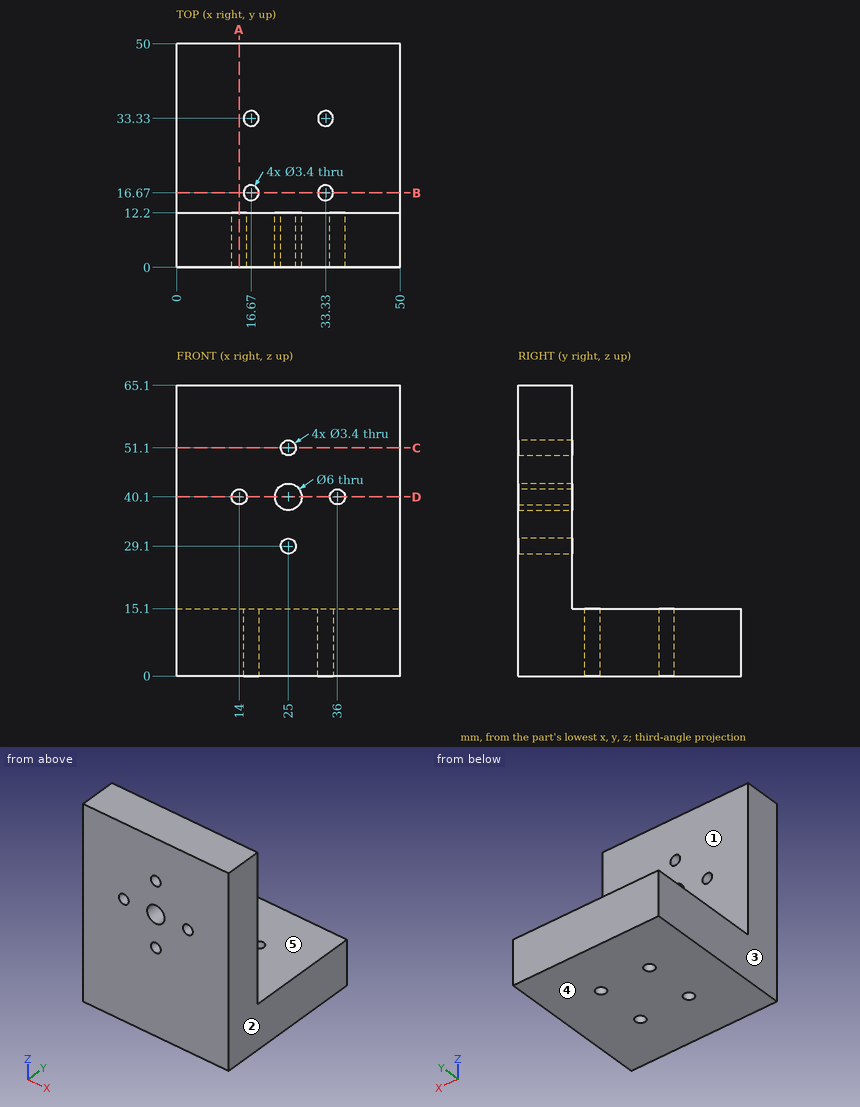
Geometry check sheet. Reference: drawing and pictorial views, mm from the part's lowest x, y, z. A direction names the side the tool comes from. Coordinates: 2 decimals unless noted, no trailing zeros. Write each loop counter-clockwise with the first axis right and the second up, starting at its lowest first coordinate (ties: lowest second). Pieces come first, ordered by that corner, then holes. Notation, with made-up numbers: (81.25, 37.25) -> (87.25, 37.25) arc R24 ccw to (87.25, 51.25) -> close; hole circle Ø8 at (63, 33). An arc over 180 degrees is marked (long way). Use a Markdown table: item, result.
1. Sectioned sample at D-D (z = 40.1). Enter the section's corners in (x, y), plus the area to 3 significant figures.
Reported:
| item | result |
|---|---|
| outline | (0, 0) -> (12.3, 0) -> (12.3, 12.2) -> (0, 12.2) -> close; (15.7, 0) -> (22, 0) -> (22, 12.2) -> (15.7, 12.2) -> close; (28, 0) -> (34.3, 0) -> (34.3, 12.2) -> (28, 12.2) -> close; (37.7, 0) -> (50, 0) -> (50, 12.2) -> (37.7, 12.2) -> close |
| area | 454 mm2 |
2. Sectioned sample at A-A (x = 14). Enter the section's corners in (y, z).
Reported:
| item | result |
|---|---|
| outline | (0, 0) -> (50, 0) -> (50, 15.1) -> (12.2, 15.1) -> (12.2, 38.4) -> (0, 38.4) -> close; (0, 41.8) -> (12.2, 41.8) -> (12.2, 65.1) -> (0, 65.1) -> close |
3. Sectioned sample at B-B (y = 16.67). Enter the section's corners in (x, z), plus the area to 3 significant figures.
Reported:
| item | result |
|---|---|
| outline | (0, 0) -> (14.97, 0) -> (14.97, 15.1) -> (0, 15.1) -> close; (18.37, 0) -> (31.63, 0) -> (31.63, 15.1) -> (18.37, 15.1) -> close; (35.03, 0) -> (50, 0) -> (50, 15.1) -> (35.03, 15.1) -> close |
| area | 652 mm2 |
4. Sectioned sample at C-C (z = 51.1). Enter the section's corners in (x, y), plus the area to 3 significant figures.
Reported:
| item | result |
|---|---|
| outline | (0, 0) -> (23.3, 0) -> (23.3, 12.2) -> (0, 12.2) -> close; (26.7, 0) -> (50, 0) -> (50, 12.2) -> (26.7, 12.2) -> close |
| area | 569 mm2 |
5. Tool access check on the marked faces 4 and 5. Record the directions out of +Z, -Z, +X, -X, +Y, -Y that give a thin tool (end or side, any length) a straight path to the whole face; none if there is none.
Reported:
| item | result |
|---|---|
| face 4 | -Z, +X, -X, +Y, -Y |
| face 5 | +Z, +X, -X, +Y |
6. Release check for a two-part mould opening along X. For the marked faces 1, 2 and 3 record: pulls with the +X half, pulls with the -X half, needs draft (parallel to the pull), parting line crosses it, or undercut.
Reported:
| item | result |
|---|---|
| face 1 | needs draft |
| face 2 | pulls with the +X half |
| face 3 | pulls with the -X half |
7. Go/stop test with flat-tipped pins: pin 1 Ø6 at (y, z) = (14, 53) entering from -X; pin 2 Ø4.5 at (x, z) = (25, 51.1) entering from +Y. Record where each tip stops, or that it passes through.
Reported:
| item | result |
|---|---|
| pin 1 | stops at x = 0 |
| pin 2 | stops at y = 12.2 |
8. Scan lines: line 1 along Y through (x, z) = (16.67, 10); line 2 along X through (y, z) = (4, 40); line 3 along X through (y, z) = (33, 10). Record each from-to range of solid material in increasing order.
Reported:
| item | result |
|---|---|
| line 1 | y = 0 to 14.97, 18.37 to 31.63, 35.03 to 50 |
| line 2 | x = 0 to 12.3, 15.7 to 22, 28 to 34.3, 37.7 to 50 |
| line 3 | x = 0 to 15, 18.34 to 31.66, 35 to 50 |
